from build123d import *

# Parameters (mm, degrees)
F0_W      = 69.954097271
F0_H      = 109.3032807112
F0_W_2    = 60.0439347327
F0_H_2    = 102.8908193111
F1_DEPTH  = 6.604
F2_R      = 5.08
F3_R      = 5.08
F4_R      = 5.08
F5_R      = 5.08
F7_R      = 4.5439536935
F8_DEPTH  = 5.08
F6_W      = 54.8973716795
F6_H      = 85.8501419425
F10_DEPTH = 0.762
F9_R      = 4.2471129498
F11_DEPTH = 0.508
F12_W     = 11.9684562087
F12_H     = 3.1413002871
F13_DEPTH = 27.432
F14_W     = 9.9000707269
F14_H     = 2.8742142022
F15_DEPTH = 36.068
F16_W     = 8.7329447269
F16_H     = 1.5476101544
F17_DEPTH = 35.56
F18_W     = 8.8735893369
F18_H     = 2.9995241202
F20_DEPTH = 35.814
F19_W     = 8.1237098202
F19_H     = 2.9995241202
F21_DEPTH = 35.814
F22_W     = 7.1957183536
F22_H     = 1.4391434379
F23_DEPTH = 54.61
F24_R     = 4.8808100994
F25_DEPTH = 6.858
F26_W     = 13.9698619023
F26_H     = 2.2988393903
F27_DEPTH = 0.762


with BuildPart() as f1:
    # F0 (on Top) → F1 (new body)
    with BuildSketch(Plane.XY):
        Rectangle(F0_W, F0_H)
        Rectangle(F0_W_2, F0_H_2, mode=Mode.SUBTRACT)
        Rectangle(F0_W_2, F0_H_2)
    extrude(amount=F1_DEPTH)

    # F2
    f2_edges = [f1.edges().sort_by_distance(p)[0] for p in [
        (34.977049, -54.65164, 3.302),
    ]]
    fillet(f2_edges, radius=F2_R)

    # F3
    f3_edges = [f1.edges().sort_by_distance(p)[0] for p in [
        (-34.977049, -54.65164, 3.302),
    ]]
    fillet(f3_edges, radius=F3_R)

    # F4
    f4_edges = [f1.edges().sort_by_distance(p)[0] for p in [
        (34.977049, 54.65164, 3.302),
    ]]
    fillet(f4_edges, radius=F4_R)

    # F5
    f5_edges = [f1.edges().sort_by_distance(p)[0] for p in [
        (-34.977049, 54.65164, 3.302),
    ]]
    fillet(f5_edges, radius=F5_R)

    # F7 (on Top) → F8 (join)
    with BuildSketch(Plane.XY):
        with Locations((0, -49.0902625024)):
            Circle(F7_R)
    extrude(amount=F8_DEPTH)

    # F6 (on Top) → F10 (join)
    with BuildSketch(Plane.XY):
        Rectangle(F6_W, F6_H)
    extrude(amount=-F10_DEPTH)

    # F9 (on Top) → F11 (join)
    with BuildSketch(Plane.XY):
        with Locations((0, -49.5532862842)):
            Circle(F9_R)
    extrude(amount=-F11_DEPTH)

    # F12 (on Right) → F13 (join)
    with BuildSketch(Plane.YZ):
        with Locations((37.5296398997, 3.3532099333)):
            Rectangle(F12_W, F12_H)
    extrude(amount=F13_DEPTH)

    # F14 (on Right) → F15 (join)
    with BuildSketch(Plane.YZ):
        with Locations((37.1129624546, 2.9665301554)):
            Rectangle(F14_W, F14_H)
    extrude(amount=-F15_DEPTH)

    # F16 (on Right) → F17 (join)
    with BuildSketch(Plane.YZ):
        with Locations((37.7242527902, 3.5489225993)):
            Rectangle(F16_W, F16_H)
    extrude(amount=F17_DEPTH)

    # F18 (on Right) → F20 (join)
    with BuildSketch(Plane.YZ):
        with Locations((26.1136516929, 3.4715009388)):
            Rectangle(F18_W, F18_H)
    extrude(amount=F20_DEPTH)

    # F19 (on Right) → F21 (join)
    with BuildSketch(Plane.YZ):
        with Locations((15.2403791435, 3.4715009388)):
            Rectangle(F19_W, F19_H)
    extrude(amount=F21_DEPTH)

    # F22 (on Front) → F23 (join)
    with BuildSketch(Plane.XZ):
        with Locations((-0.2988093765, 3.7136741448)):
            Rectangle(F22_W, F22_H)
    extrude(amount=F23_DEPTH)

    # F24 (on Top) → F25 (join)
    with BuildSketch(Plane.XY):
        with Locations((-25.2635255456, 43.6428338289)):
            Circle(F24_R)
    extrude(amount=F25_DEPTH)

    # F26 (on Top) → F27 (join)
    with BuildSketch(Plane.XY):
        with Locations((-0.0951243564, 47.2962372005)):
            Rectangle(F26_W, F26_H)
    extrude(amount=-F27_DEPTH)


solid = f1.part
Can you work these out from the model? Positions are in its coordinate system, mm. A direction names the side the tool comes from. Coordinates: 2 decimals unless noted, no trailing zeros. Write each loop counter-clockwise with the first axis right and the second up, starting at its lowest first coordinate (ties: lowest second). Pieces come first, ordered by that corner, then holes. Notation, with made-up numbers: (45.5, 15) -> (58.5, 15) arc R9 cw to (58.5, 23) -> close; hole circle Ø1 at (70.25, 31.5). An arc over 180 degrees is marked (long way). Answer as CSV lines item,"result".
1) If we mould it in two halves opening along Y, with no side actions, what happens to faces 1 (the flat face through (35.814, 26, 3)), 2 (the cylindrical face through (-33.45, 53.2, 3.35)), 3 (the cylindrical face through (2, -53.3, -0.3))? For each: +Y half, -Y half, draft (parallel to the pull), parting line (faces both ways), or undercut.
Check result:
face 1,"draft"
face 2,"+Y half"
face 3,"undercut"
2) Will these pins go through, and if not, where does the flat tip stop? P1, Ø0.7, axis at x = 35.5, y = 14.5, coming from the +Z side; P2, Ø0.5, axis at x = -35.5, z = 3, coming from the -Y side; P3, Ø2, axis at x = -19.5, y = -12, coming from the +Z side.
Check result:
P1,"z = 4.97"
P2,"y = 32.16"
P3,"z = 6.6"
3) On a 3-axis mill with a long thin cutter (end or side, diameter ignored), from which of +Z, -Z, +X, -X, +Y, -Y can I reach the whole of each face in a straight line? I mean faces 4 (the flat face through (35.814, 15, 3)), 5 (the flat face through (0, -49, -0.508)). Say none if no direction works.
Check result:
face 4,"+Z, -Z, +X, +Y, -Y"
face 5,"-Z, +X, -X, -Y"
4) If we section it at A-A on y = -31: Please give me the cut outline in (x, z), then the cut area to 3 significant figures.
Check result:
outline,"(-34.98, 0) -> (-27.45, 0) -> (-27.45, -0.76) -> (27.45, -0.76) -> (27.45, 0) -> (34.98, 0) -> (34.98, 6.6) -> (-34.98, 6.6) -> close"
area,"504 mm²"
5) If we section it at C-C on x = 0: Please give me the cut outline in (y, z).
Check result:
outline,"(-54.65, 0) -> (-53.8, 0) -> (-53.8, -0.51) -> (-45.31, -0.51) -> (-45.31, 0) -> (-42.93, 0) -> (-42.93, -0.76) -> (42.93, -0.76) -> (42.93, 0) -> (46.15, 0) -> (46.15, -0.76) -> (48.45, -0.76) -> (48.45, 0) -> (54.65, 0) -> (54.65, 6.6) -> (-54.65, 6.6) -> close"
6) If I drill on line 1 (Z direction, x = 9, y = -21.5); line 2 (X direction, y = -13.5, z = 1.25); line 3 (X direction, y = 29.5, z = 3.5), over which ranges is the centre line in solid material (lowest first)? Write a range as from..to.
Check result:
line 1,"-0.76..6.6"
line 2,"-34.98..34.98"
line 3,"-34.98..35.81"
7) If we section it at B-B on x = -19: Please give me the cut outline in (y, z).
Check result:
outline,"(-54.65, 0) -> (-42.93, 0) -> (-42.93, -0.76) -> (42.93, -0.76) -> (42.93, 0) -> (54.65, 0) -> (54.65, 6.6) -> (-54.65, 6.6) -> close"
